```python
from build123d import *

# Parameters (mm, degrees)
F1_DEPTH = 812
F2_R     = 2.5
F3_DEPTH = 10.001
F4_R     = 2.5
F5_DEPTH = 25.001


with BuildPart() as f1:
    # F0 (on Top) → F1 (new body)
    with BuildSketch(Plane.XY):
        Polygon((-28.650518, 0), (-238.650518, 0), (-238.650518, -25), (261.349482, -25), (261.349482, 0), (51.349482, 0), (51.349482, -15), (-28.650518, -15), align=None)
    extrude(amount=F1_DEPTH)

    # F2 (on face) → F3 (cut, through all)
    with BuildSketch(Plane(origin=(0, -15, 0), x_dir=(-1, 0, 0), z_dir=(0, 1, 0))):
        with Locations((-11.349482, 406)):
            Circle(F2_R)
    extrude(amount=-F3_DEPTH, mode=Mode.SUBTRACT)

    # F4 (on face) → F5 (cut, through all)
    with BuildSketch(Plane.XZ.offset(25)):
        with Locations((11.349482, 452)):
            Circle(F4_R)
    extrude(amount=-F5_DEPTH, mode=Mode.SUBTRACT)


solid = f1.part
```
Here's how the part is built. I have some questions about the finished solid (model axes, mm). A direction names the side the tool comes from. Coordinates: 2 decimals unless noted, no trailing zeros. Loops run counter-clockwise (first coordinate to the right, second up) from the corner with the lowest first, then second, coordinate; pieces in that order, holes last. Notation, with made-up numbers: (36, 24.25) -> (79, 24.25) arc R12 cw to (79, 36.25) -> close; hole circle Ø2 at (-22, 71.5). An arc over 180 degrees is marked (long way). Return JSON: item names as keys, results as strings.
1) For faces 1 (the face through (-28.651, -8, 400)), 2 (the face through (-238.651, -12, 400)), which set-ups out of +Z, -Z, +X, -X, +Y, -Y let a thin tool reach every point of the face, with its end or its side?
Results below:
{"face 1": "+Z, -Z, +Y", "face 2": "+Z, -Z, -X, +Y, -Y"}
2) If we section it at B-B, the plane z = 142: Write out the boundary of the cut face in (x, y), then the cut area to 3 significant figures.
Results below:
{"outline": "(-238.65, -25) -> (261.35, -25) -> (261.35, 0) -> (51.35, 0) -> (51.35, -15) -> (-28.65, -15) -> (-28.65, 0) -> (-238.65, 0) -> close", "area": "11,300 mm²"}
3) Thinking about a two-plate mould opening in X: for faces 3 (the face through (261.349, -13, 400)), 4 (the face through (8, -18, 0)), 5 (the face through (51.349, -7, 400)), which applies, +X half, -X half, draft (parallel to the pull), parting line (faces both ways), or undercut?
Results below:
{"face 3": "+X half", "face 4": "draft", "face 5": "undercut"}
4) If we section it at A-A, the plane y = -5.75: Write out the boundary of the cut face in (x, z), then the cut area to 3 significant figures.
Results below:
{"outline": "(-238.65, 0) -> (-28.65, 0) -> (-28.65, 812) -> (-238.65, 812) -> close; (51.35, 0) -> (261.35, 0) -> (261.35, 812) -> (51.35, 812) -> close", "area": "341,000 mm²"}
5) I need wall thicknesses on line 1 (X direction, y = -18, z = 406); line 2 (X direction, y = -9, z = 292.5). Which ranges of each line are inside material? Lowest first, please. Write a range as from..to.
Results below:
{"line 1": "-238.65..8.85, 13.85..261.35", "line 2": "-238.65..-28.65, 51.35..261.35"}
6) Will this pin go through, and if not, where does the flat tip stop? pin 1 (4 mm diameter, centred on x = 11.35, z = 406, fed in from -Y).
Results below:
{"pin 1": "through"}
